Design review of the part built by this model. Coordinates are the model's own, in mm. Coordinates: 2 decimals unless noted, no trailing zeros. Loops run counter-clockwise (first coordinate to the right, second up) from the corner with the lowest first, then second, coordinate; pieces in that order, holes last.
Q1. Add section C-C on z = -10. Give the boundary of the cut face in (x, y) (3 decimals), and give its area (3 significant figures).
Q2. Add section A-A on x = 10.5. Give the boundary of the cut face in (y, z) (3 decimals).
Q3. Wall thickness on probe 1 along Z at (x, y) = (139.5, 2.35) (3 decimals); probe 2 along X at (y, z) = (1.1, -60) (3 decimals); probe 3 along X at (y, z) = (1.4, -58): over which ranges is each line inside the solid? List them lowest first.
Q4. For P1, Ø5.5, axis at x = 139.5, z = -10, coming from the +Y side, flat-tipped, find the tip position at first contact; note if it passes through.
Q5. Add section D-D on x = 139.5. Give the boundary of the cut face in (y, z) (3 decimals), and give its area (3 significant figures).
Q6. Add section B-B on y = 1.45. Give the boundary of the cut face in (x, z) (3 decimals).
Q7. Draft analysis for pull direction X (two halves, no side actions). For faces 1 (the face through (8.202, 1.521, -29.984)), 2 (the face through (74, 1, -70)), 3 (the face through (142.65, 1.52, -10.41)), 4 (the face through (147.745, 1.521, -2.139)), state which applies: released by +X, released by -X, zero draft, split by the parting line, or undercut.
```python
from build123d import *

# Parameters (mm, degrees)
ESBO_O2_W                = 150
ESBO_O2_H                = 70
RESSALTO_EXTRUS_O1_DEPTH = 3
ESBO_O4_R                = 3.175
CORTE_EXTRUS_O1_DEPTH    = 3
FILETE1_R                = 7.5
ESBO_O6_R                = 6
CORTE_EXTRUS_O2_DEPTH    = 10


with BuildPart() as part:
    # Esboço2 → Ressalto-extrusão1 (new body)
    with BuildSketch(Plane(origin=(0, 0, 0), x_dir=(1, 0, 0), z_dir=(0, 1, 0))):
        with Locations((75, 35)):
            Rectangle(ESBO_O2_W, ESBO_O2_H)
    extrude(amount=RESSALTO_EXTRUS_O1_DEPTH)

    # Esboço4 → Corte-extrusão1 (cut)
    with BuildSketch(Plane(origin=(0, 3, 0), x_dir=(1, 0, 0), z_dir=(0, 1, 0))):
        with Locations(Location((10.5, 60, 0), (0, 0, 270))):
            Circle(ESBO_O4_R)
        with Locations(Location((139.5, 60, 0), (0, 0, 270))):
            Circle(ESBO_O4_R)
        with Locations(Location((139.5, 10, 0), (0, 0, 270))):
            Circle(ESBO_O4_R)
        with Locations(Location((10.5, 10, 0), (0, 0, 270))):
            Circle(ESBO_O4_R)
    extrude(amount=-CORTE_EXTRUS_O1_DEPTH, mode=Mode.SUBTRACT)

    # Filete1
    filete1_edges = [part.edges().sort_by_distance(p)[0] for p in [
        (0, 1.5, -70),
        (150, 1.5, -70),
        (150, 1.5, 0),
        (0, 1.5, 0),
    ]]
    fillet(filete1_edges, radius=FILETE1_R)

    # Esboço6 → Corte-extrusão2 (cut)
    with BuildSketch(Plane(origin=(0, 3, 0), x_dir=(1, 0, 0), z_dir=(0, 1, 0))):
        with Locations(Location((10.5, 35.526964124, 0), (0, 0, 270))):
            Circle(ESBO_O6_R)
    extrude(amount=-CORTE_EXTRUS_O2_DEPTH, mode=Mode.SUBTRACT)


solid = part.part
```
Entries:
1. outline: (0, 0) - (7.325, 0) - (7.325, 3) - (0, 3) - close; (13.675, 0) - (136.325, 0) - (136.325, 3) - (13.675, 3) - close; (142.675, 0) - (150, 0) - (150, 3) - (142.675, 3) - close
1. area: 412 mm2
2. outline: (0, -70) - (3, -70) - (3, -63.175) - (0, -63.175) - close; (0, -56.825) - (3, -56.825) - (3, -41.527) - (0, -41.527) - close; (0, -29.527) - (3, -29.527) - (3, -13.175) - (0, -13.175) - close; (0, -6.825) - (3, -6.825) - (3, 0) - (0, 0) - close
3. probe 1: z = -70 to -63.175, -56.825 to -13.175, -6.825 to 0
3. probe 2: x = 0 to 7.325, 13.675 to 136.325, 142.675 to 150
3. probe 3: x = 0 to 8.03, 12.97 to 137.03, 141.97 to 150
4. P1: passes through
5. outline: (0, -70) - (3, -70) - (3, -63.175) - (0, -63.175) - close; (0, -56.825) - (3, -56.825) - (3, -13.175) - (0, -13.175) - close; (0, -6.825) - (3, -6.825) - (3, 0) - (0, 0) - close
5. area: 172 mm2
6. outline: (0, -62.5) arc R7.5 ccw to (7.5, -70) - (142.5, -70) arc R7.5 ccw to (150, -62.5) - (150, -7.5) arc R7.5 ccw to (142.5, 0) - (7.5, 0) arc R7.5 ccw to (0, -7.5) - close; hole circle Ø12 at (10.5, -35.527); hole circle Ø6.35 at (10.5, -60); hole circle Ø6.35 at (10.5, -10); hole circle Ø6.35 at (139.5, -60); hole circle Ø6.35 at (139.5, -10)
7. face 1: undercut
7. face 2: zero draft
7. face 3: undercut
7. face 4: released by +X
